Here's how the part is built. I have some questions about the finished solid (model axes, mm). Face numbers are marked on the shaded views. A direction names the side the tool comes from. Round coordinates to 2 decimals unless told otherwise and drop trailing zeros. Loops run counter-clockwise (first coordinate to the right, second up) from the corner with the lowest first, then second, coordinate; pieces in that order, holes last. Notation, with made-up numbers: M 84,65 L 133,65 A35 ccw 133,99 Z; hole C -22.5,16 d10. An arc over 180 degrees is marked long. Answer as CSV lines item,"result".
```python
from build123d import *

# Parameters (mm, degrees)
F2_W     = 4.7625
F2_H     = 4.7625
F3_DEPTH = 86.51975


with BuildPart() as f1:
    # F0 (on Front) → F1 (revolve)
    with BuildSketch(Plane.XZ):
        Polygon((0, 107.95), (0, 9.525), (86.51875, 9.525), (86.51875, 28.575), (83.34375, 35.383809), (83.34375, 46.0375), (32.54375, 46.0375), (32.54375, 107.95), (31.050549, 107.95), (27.384375, 101.6), (5.159375, 101.6), (1.493201, 107.95), align=None)
    revolve(axis=Axis((43.259375, 0, 0), (1, 0, 0)))

    # F2 (on Right) → F3 (cut, through all)
    with BuildSketch(Plane.YZ):
        with Locations((0, 9.21385)):
            Rectangle(F2_W, F2_H)
    extrude(amount=F3_DEPTH, mode=Mode.SUBTRACT)


solid = f1.part
```
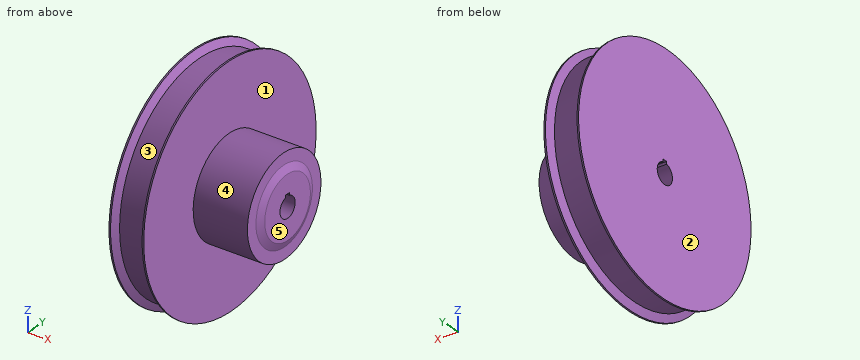
1. Which directions (+Z, -Z, +X, -X, +Y, -Y) give clear straight access to the entire face, cutting with the end or side of a thin tool? Please do the marked faces 4 and 5.
Evaluation:
face 4,"+X"
face 5,"+Z, -Z, +X, +Y, -Y"
2. We'd pull the mould along X, two halves only. Please class the marked faces 1, 2 and 3: pulls with the +X half, pulls with the -X half, needs draft (parallel to the pull), parting line crosses it, or undercut.
Evaluation:
face 1,"pulls with the +X half"
face 2,"pulls with the -X half"
face 3,"undercut"
3. I want a section at C-C, the plane x = 11.5. Please give me the cut outline in (y, z) (3 decimals), and give its area (3 significant figures).
Evaluation:
outline,"C 0,0 d203.2; hole M -2.381,9.223 A9.525 ccw long 2.381,9.223 L 2.381,11.595 L -2.381,11.595 Z"
area,"32,100 mm²"
4. If I drill on line 1 (Z direction, x = 49, y = 0) (1 decimal); line 2 (Y direction, x = 34, z = 0) (1 decimal); line 3 (X direction, y = -36, z = 22), over which ranges is the centre line in solid material (lowest first)? Write a range as [from, to].
Evaluation:
line 1,"z = [-46, -9.5], [11.6, 46]"
line 2,"y = [-46, -9.5], [9.5, 46]"
line 3,"x = [0, 83.34]"
5. For P1, Ø2.5, axis at x = 62.5, z = 10.5, coming from the -Y side; P2, Ø8, axis at x = 19.5, y = 71.5, coming from the -Z side; P3, Ø5, axis at x = 30, y = -48.5, coming from the +Z side, each with a flat end and sliding along its axis, tell me the tip position at first contact or that it passes through.
Evaluation:
P1,"stops at y = -45.1"
P2,"stops at z = -75.94"
P3,"stops at z = 97.55"
